The drawing under review shows one solid part. Ordinate dimensions are in mm from its lowest x, y, z. A direction names the side the tool comes from. Coordinates: 2 decimals unless noted, no trailing zeros. Loops run counter-clockwise (first coordinate to the right, second up) from the corner with the lowest first, then second, coordinate; pieces in that order, holes last. Notation, with made-up numbers: (-5, 36.25) - (41, 36.25) arc R30 cw to (41, 69.25) - close; hole circle Ø4 at (16.25, 4). An arc over 180 degrees is marked (long way). Answer as a JSON object with one key per item and string values. Group by question number.
Item 1: Clearance check with flat-ended pins moving along their axes: pin 1 (1.2 mm diameter, centred on x = 16, y = 2.5, fed in from +Z); pin 2 (1.4 mm diameter, centred on y = 24.82, z = 2.21, fed in from +X) (3 decimals). State where each tip first meets the part, or that it passes through.
Item 2: We need section B-B (y = 6.5). Give the boundary of the cut face in (x, z) (1 decimal).
Item 3: We need section C-C (z = 2.8). Give the boundary of the cut face in (x, y) (1 decimal).
Item 4: Mouldability with a two-part tool opening along Y and no side actions: class the marked faces 3, 4, 5 and 6 as released by +Y, released by -Y, zero draft, split by the parting line, or undercut.
Item 5: Tool access review of the marked faces 1 and 2: name each direction out of +Z, -Z, +X, -X, +Y, -Y from which nothing blocks a thin tool from reaching the whole face with its end or side.
Item 6: To check wall thickness, follow line 1 (Y direction, x = 12.25, z = 3.15) (1 decimal); line 2 (Y direction, x = 21.5, z = 0.8) (1 decimal); line 3 (X direction, y = 19, z = 2.7) (1 decimal). State the ranges of each line that lie inside material, in increasing order.
Item 7: We need section D-D (y = 15). Give the boundary of the cut face in (x, z) (1 decimal).
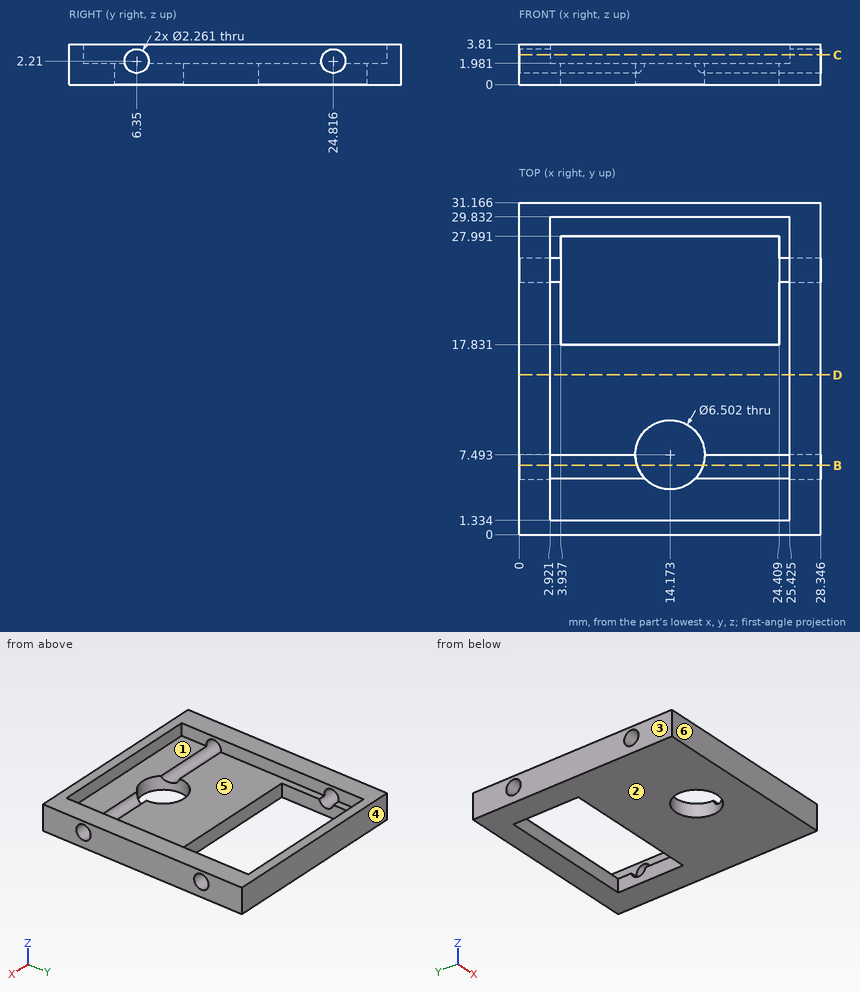
Check sheet entries:
{
 "1": {"pin 1": "stops at z = 1.98", "pin 2": "passes through"},
 "2": {"outline": "(0, 0) - (11.1, 0) - (11.1, 1.1) - (0, 1.1) - close; (0, 3.3) - (2.9, 3.3) - (2.9, 3.8) - (0, 3.8) - close; (17.3, 0) - (28.3, 0) - (28.3, 1.1) - (17.3, 1.1) - close; (25.4, 3.3) - (28.3, 3.3) - (28.3, 3.8) - (25.4, 3.8) - close"},
 "3": {"outline": "(0, 0) - (28.3, 0) - (28.3, 5.4) - (25.4, 5.4) - (25.4, 1.3) - (2.9, 1.3) - (2.9, 5.4) - (0, 5.4) - close; (0, 7.3) - (2.9, 7.3) - (2.9, 23.9) - (0, 23.9) - close; (0, 25.8) - (2.9, 25.8) - (2.9, 29.8) - (25.4, 29.8) - (25.4, 25.8) - (28.3, 25.8) - (28.3, 31.2) - (0, 31.2) - close; (25.4, 7.3) - (28.3, 7.3) - (28.3, 23.9) - (25.4, 23.9) - close"},
 "4": {"face 3": "zero draft", "face 4": "released by +Y", "face 5": "undercut", "face 6": "released by -Y"},
 "5": {"face 1": "+Z", "face 2": "-Z, +X, -X, +Y, -Y"},
 "6": {"line 1": "y = 0 to 1.3, 29.8 to 31.2", "line 2": "y = 0 to 17.8, 28 to 31.2", "line 3": "x = 0 to 2.9, 25.4 to 28.3"},
 "7": {"outline": "(0, 0) - (28.3, 0) - (28.3, 3.8) - (25.4, 3.8) - (25.4, 2) - (2.9, 2) - (2.9, 3.8) - (0, 3.8) - close"}
}
